Read the model definition and answer for the solid it produces. Units are mm, in the model's axes. A direction names the side the tool comes from. Give positions to 0.01 mm unless a question says otherwise; leave off trailing zeros. Write each loop counter-clockwise with the first axis right and the second up, starting at its lowest first coordinate (ties: lowest second). Pieces come first, ordered by that corner, then holes. Notation, with made-up numbers: M 47.5,77 L 67.5,77 A29 cw 67.5,113 Z; hole C -20.75,-22.75 d6. An arc over 180 degrees is marked long. Use a Markdown table: item, result. Add a question column.
Item 1: Consider probe 1 along Y at (x, z) = (-27.5, -0.85); probe 2 along Y at (x, z) = (-8, 0); probe 3 along X at (y, z) = (-8, -0.55). Determine where each line is inside the solid, lowest interval first. Write a range as [from, to].
Item 2: A cutting plane is placed at C-C on y = 3.5. Determine the outline of the cut face in (x, z).
Item 3: Given P1, Ø1, axis at x = -1.5, z = 0, coming from the -Y side, flat-ended and moving along its own axis, determine where the tip first touches the part or whether it passes through.
Item 4: The mould has two halves that part along X. Classify faces 3 (the flat face through (54, -1, 0)), 4 (the flat face through (8.9, -36.4, 0)), 5 (the flat face through (-9, -36.5, 0)), 6 (the flat face through (-1, 9, 1.588)): pulls with the +X half, pulls with the -X half, needs draft (parallel to the pull), parting line crosses it, or undercut.
Item 5: For faces 1 (the cylindrical face through (-0.911, 4.615, 0.022)), 2 (the cylindrical face through (5.76, -33.98, -0.02)), determine the directions among +Z, -Z, +X, -X, +Y, -Y from which every point of the face is accessible in a straight line to the end or side of a thin tool.
Item 6: A cutting plane is placed at B-B on x = 16.5. Determine the outline of the cut face in (y, z), then the cut area to 3 significant figures.
Item 7: A cutting plane is placed at A-A on y = -25.5. Determine the outline of the cut face in (x, z), then the cut area to 3 significant figures.
Item 8: A cutting plane is placed at D-D on z = 1.05. Determine the outline of the cut face in (x, y) (3 decimals).
Autodesk Inventor part; units mm, degrees
ref_plane "YZ Plane" through (0, 0, 0) normal (1, 0, 0) x (0, 1, 0)
ref_plane "XZ Plane" through (0, 0, 0) normal (0, 1, 0) x (-1, 0, 0)
ref_plane "XY Plane" through (0, 0, 0) normal (0, 0, 1) x (1, 0, 0)
sketch "Sketch1" plane through (0, 0, 0) normal (0, 0, 1) x (1, 0, 0)
  line L0 (-54, -37.5) -> (54, -37.5)
  line L1 (54, -37.5) -> (54, 37.5)
  line L2 (54, 37.5) -> (-54, 37.5)
  line L3 (-54, 37.5) -> (-54, -37.5)
  line L4 (-54, -37.5) -> (54, 37.5) construction
  line L5 (54, -37.5) -> (-54, 37.5) construction
  point P0 (0, 0)
  dimension "d0" = 108
  dimension "d1" = 75
extrude "Extrusion1" add sketch "Sketch1" along normal mid plane 3.175
sketch "Sketch3" plane through (0, 0, 1.5875) normal (0, 0, 1) x (1, 0, 0)
  line L0 (-54, -37.5) -> (54, -37.5) construction
  line L1 (-10, -37.5) -> (-6, -33.5)
  line L2 (-6, -33.5) -> (6, -33.5)
  line L3 (6, -33.5) -> (10, -37.5)
  line L4 (-10, -37.5) -> (10, -37.5)
  point P0 (0, 0)
  point P1 (0, -33.5)
  point P2 (0, -37.5)
  dimension "d16" = 12
  dimension "d17" = 4
  dimension "d18" = 45
extrude "Extrusion3" cut sketch "Sketch3" against normal through all
fillet "Fillet1" radius 6.5 2 edges at (-6, -33.5, 0) (6, -33.5, 0)
sketch "Sketch4" plane through (0, 0, 1.5875) normal (0, 0, 1) x (1, 0, 0)
  circle A0 centre (0, -2.325) radius 7
  line L0 (10, -37.5) -> (54, -37.5) construction
  point P0 (0, 0)
  dimension "d22" = 14
  dimension "d23" = 35.175
extrude "Extrusion4" cut sketch "Sketch4" against normal through all
sketch "Sketch5" plane through (0, 0, 1.5875) normal (0, 0, 1) x (1, 0, 0)
  circle A0 centre (-27.5, -25.5) radius 3
  line L0 (-54, -37.5) -> (-10, -37.5) construction
  circle A1 centre (-16.5, -25.5) radius 3
  circle A2 centre (-5.5, -25.5) radius 3
  circle A3 centre (5.5, -25.5) radius 3
  circle A4 centre (16.5, -25.5) radius 3
  circle A5 centre (27.5, -25.5) radius 3
  line L1 (-5.5, -25.5) -> (5.5, -25.5) construction
  point P0 (0, 0)
  point P1 (0, -25.5)
  dimension "d26" = 6
  dimension "d27" = 12
  dimension "d30" = 11
extrude "Extrusion5" cut sketch "Sketch5" against normal blind 10
properties part number "ArmSupportPlate"
Filled in:
| question | item | result |
|---|---|---|
| 1 | probe 1 | [-37.5, -28.5], [-22.5, 37.5] |
| 1 | probe 2 | [-35.5, -27.16], [-23.84, 37.5] |
| 1 | probe 3 | [-54, -4.1], [4.1, 54] |
| 2 | outline | M -54,-1.59 L -3.88,-1.59 L -3.88,1.59 L -54,1.59 Z; M 3.88,-1.59 L 54,-1.59 L 54,1.59 L 3.88,1.59 Z |
| 3 | P1 | y = -33.5 |
| 4 | face 3 | pulls with the +X half |
| 4 | face 4 | undercut |
| 4 | face 5 | undercut |
| 4 | face 6 | needs draft |
| 5 | face 1 | +Z, -Z |
| 5 | face 2 | +Z, -Z, -Y |
| 6 | outline | M -37.5,-1.59 L -28.5,-1.59 L -28.5,1.59 L -37.5,1.59 Z; M -22.5,-1.59 L 37.5,-1.59 L 37.5,1.59 L -22.5,1.59 Z |
| 6 | area | 219 mm² |
| 7 | outline | M -54,-1.59 L -30.5,-1.59 L -30.5,1.59 L -54,1.59 Z; M -24.5,-1.59 L -19.5,-1.59 L -19.5,1.59 L -24.5,1.59 Z; M -13.5,-1.59 L -8.5,-1.59 L -8.5,1.59 L -13.5,1.59 Z; M -2.5,-1.59 L 2.5,-1.59 L 2.5,1.59 L -2.5,1.59 Z; M 8.5,-1.59 L 13.5,-1.59 L 13.5,1.59 L 8.5,1.59 Z; M 19.5,-1.59 L 24.5,-1.59 L 24.5,1.59 L 19.5,1.59 Z; M 30.5,-1.59 L 54,-1.59 L 54,1.59 L 30.5,1.59 Z |
| 7 | area | 229 mm² |
| 8 | outline | M -54,-37.5 L -10,-37.5 L -7.904,-35.404 A6.5 cw -3.308,-33.5 L 3.308,-33.5 A6.5 cw 7.904,-35.404 L 10,-37.5 L 54,-37.5 L 54,37.5 L -54,37.5 Z; hole C -27.5,-25.5 d6; hole C -16.5,-25.5 d6; hole C -5.5,-25.5 d6; hole C 0,-2.325 d14; hole C 5.5,-25.5 d6; hole C 16.5,-25.5 d6; hole C 27.5,-25.5 d6 |
